Geometry: final body of the model. Coordinates: model frame, mm. Face numbers are marked on the shaded views. A direction names the side the tool comes from. Round coordinates to 2 decimals unless told otherwise and drop trailing zeros. Loops run counter-clockwise (first coordinate to the right, second up) from the corner with the lowest first, then second, coordinate; pieces in that order, holes last. Notation, with made-up numbers: M 60.25,-21.75 L 109.25,-21.75 A17 cw 109.25,-5.75 Z; hole C 63,54 d6. An arc over 180 degrees is marked long. Write each question's results on one line, items separated by ' | '.
```python
from build123d import *

# Parameters (mm, degrees)
F0_W      = 30
F0_H      = 30
F1_DEPTH  = 15
F2_R      = 4.5
F3_DEPTH  = 2
F5_R      = 3.5
F6_DEPTH  = 2
F7_R      = 3.5
F8_DEPTH  = 2
F9_R      = 3.5
F10_DEPTH = 2
F11_R     = 3.5
F12_DEPTH = 2
F13_R     = 3.5
F14_DEPTH = 2


with BuildPart() as f1:
    # F0 (on Front) → F1 (new body, symmetric)
    with BuildSketch(Plane.XZ):
        Rectangle(F0_W, F0_H)
    extrude(amount=F1_DEPTH, both=True)

    # F2 (on face) → F3 (cut)
    with BuildSketch(Plane.XZ.offset(15)):
        Circle(F2_R)
    extrude(amount=-F3_DEPTH, mode=Mode.SUBTRACT)

    # F5 (on face) → F6 (cut)
    with BuildSketch(Plane(origin=(0, 15, 0), x_dir=(-1, 0, 0), z_dir=(0, 1, 0))):
        with Locations((-7.5, 0)):
            Circle(F5_R)
        with Locations((-7.5, 9.25)):
            Circle(F5_R)
        with Locations((-7.5, -9.25)):
            Circle(F5_R)
        with Locations((7.5, 0)):
            Circle(F5_R)
        with Locations((7.5, -9.25)):
            Circle(F5_R)
        with Locations((7.5, 9.25)):
            Circle(F5_R)
    extrude(amount=-F6_DEPTH, mode=Mode.SUBTRACT)

    # F7 (on face) → F8 (cut)
    with BuildSketch(Plane.XY.offset(15)):
        with Locations((-7.5, 7.5)):
            Circle(F7_R)
        with Locations((7.5, 7.5)):
            Circle(F7_R)
        with Locations((7.5, -7.5)):
            Circle(F7_R)
        with Locations((-7.5, -7.5)):
            Circle(F7_R)
    extrude(amount=-F8_DEPTH, mode=Mode.SUBTRACT)

    # F9 (on face) → F10 (cut)
    with BuildSketch(Plane(origin=(0, 0, -15), x_dir=(1, 0, 0), z_dir=(0, 0, -1))):
        Circle(F9_R)
        with Locations((-7.5, -7.5)):
            Circle(F9_R)
        with Locations((7.5, 7.5)):
            Circle(F9_R)
    extrude(amount=-F10_DEPTH, mode=Mode.SUBTRACT)

    # F11 (on face) → F12 (cut)
    with BuildSketch(Plane.YZ.offset(15)):
        with Locations((-7.5, 7.5)):
            Circle(F11_R)
        with Locations((7.5, 7.5)):
            Circle(F11_R)
        with Locations((7.5, -7.5)):
            Circle(F11_R)
        with Locations((-7.5, -7.5)):
            Circle(F11_R)
        Circle(F11_R)
    extrude(amount=-F12_DEPTH, mode=Mode.SUBTRACT)

    # F13 (on face) → F14 (cut)
    with BuildSketch(Plane(origin=(-15, 0, 0), x_dir=(0, -1, 0), z_dir=(-1, 0, 0))):
        with Locations((-7.5, -7.5)):
            Circle(F13_R)
        with Locations((7.5, 7.5)):
            Circle(F13_R)
    extrude(amount=-F14_DEPTH, mode=Mode.SUBTRACT)


solid = f1.part
```
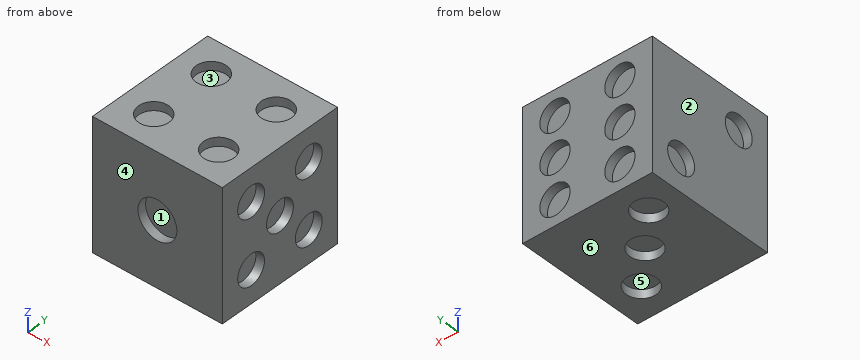
1. Pin query (flat end, axial travel): P1, Ø3.5, axis at x = 8, z = -1.5, coming from the +Y side; P2, Ø5.5, axis at x = 8.5, z = 8.5, coming from the +Y side; P3, Ø5.5, axis at x = -0.5, y = 0.5, coming from the -Z side; P4, Ø4, axis at x = 7.5, y = -7.5, coming from the +Z side. Return the tip coordinate at first contact, or that it passes through.
Answer key:
P1: stops at y = 13 | P2: stops at y = 15 | P3: stops at z = -13 | P4: stops at z = 13
2. Section C-C (y = -7.5). Output: boundary loops of the cut face in (x, z).
Answer key:
outline: M -15,-15 L 4,-15 L 4,-13 L 11,-13 L 11,-15 L 15,-15 L 15,-11 L 13,-11 L 13,-4 L 15,-4 L 15,4 L 13,4 L 13,11 L 15,11 L 15,15 L 11,15 L 11,13 L 4,13 L 4,15 L -4,15 L -4,13 L -11,13 L -11,15 L -15,15 L -15,11 L -13,11 L -13,4 L -15,4 Z
3. Section B-B (x = -7.5). Output: boundary loops of the cut face in (y, z).
Answer key:
outline: M -15,-15 L 4,-15 L 4,-13 L 11,-13 L 11,-15 L 15,-15 L 15,-12.75 L 13,-12.75 L 13,-5.75 L 15,-5.75 L 15,-3.5 L 13,-3.5 L 13,3.5 L 15,3.5 L 15,5.75 L 13,5.75 L 13,12.75 L 15,12.75 L 15,15 L 11,15 L 11,13 L 4,13 L 4,15 L -4,15 L -4,13 L -11,13 L -11,15 L -15,15 Z
4. Access query for the marked faces 1, 2 and 3. Directions: +Z, -Z, +X, -X, +Y, -Y. A direction counts if a zero-diameter tool reaches every point of the face in a straight line with its end or side. Return the directions, or none.
Answer key:
face 1: -Y | face 2: +Z, -Z, -X, +Y, -Y | face 3: +Z
5. Section D-D (x = -1.75). Output: boundary loops of the cut face in (y, z).
Answer key:
outline: M -15,-15 L -3.03,-15 L -3.03,-13 L 3.03,-13 L 3.03,-15 L 15,-15 L 15,15 L -15,15 L -15,4.15 L -13,4.15 L -13,-4.15 L -15,-4.15 Z
6. Draft query along Y for the marked faces 4, 5 and 6. Return one class per face: pulls with the +Y half, pulls with the -Y half, needs draft (parallel to the pull), parting line crosses it, or undercut.
Answer key:
face 4: pulls with the -Y half | face 5: undercut | face 6: needs draft
7. Section A-A (z = 0). Output: boundary loops of the cut face in (x, y).
Answer key:
outline: M -15,-15 L -4.5,-15 L -4.5,-13 L 4.5,-13 L 4.5,-15 L 15,-15 L 15,-3.5 L 13,-3.5 L 13,3.5 L 15,3.5 L 15,15 L 11,15 L 11,13 L 4,13 L 4,15 L -4,15 L -4,13 L -11,13 L -11,15 L -15,15 Z
8. Ray query, probe 1 along Z at (x, y) = (14.1, -7.5); probe 2 along X at (y, z) = (7.5, -13.8); probe 3 along Y at (x, z) = (-7.5, -13.8). Return the intervals inside material, ascending.
Answer key:
probe 1: z = -15 to -11, -4 to 4, 11 to 15 | probe 2: x = -15 to -11, -4 to 15 | probe 3: y = -15 to 4, 11 to 15
